Read the model definition and answer for the solid it produces. Units are mm, in the model's axes. Round coordinates to 2 decimals unless told otherwise and drop trailing zeros. Loops run counter-clockwise (first coordinate to the right, second up) from the corner with the lowest first, then second, coordinate; pieces in that order, holes last. Notation, with made-up numbers: (79.25, 5.25) -> (128.25, 5.25) arc R20 cw to (128.25, 14.25) -> close; hole circle Ø1 at (4, 11.25). An arc over 180 degrees is marked (long way). Put each result on its own line as item: value.
from build123d import *

# Parameters (mm, degrees)
BOSS_EXTRUDE1_DEPTH = 25
SKETCH2_R           = 3
CUT_EXTRUDE1_DEPTH  = 25


with BuildPart() as part:
    # Sketch1 → Boss-Extrude1 (new body, symmetric)
    with BuildSketch(Plane.XY):
        Polygon((4.75, 0), (-4.75, 0), (-11, 6.25), (-11, 7.65), (11, 7.65), (11, 6.25), align=None)
    extrude(amount=BOSS_EXTRUDE1_DEPTH, both=True)

    # Sketch2 → Cut-Extrude1 (cut, symmetric)
    with BuildSketch(Plane(origin=(0, 7.65, 0), x_dir=(1, 0, 0), z_dir=(0, 1, 0))):
        with Locations((0, 17.5)):
            Circle(SKETCH2_R)
        with Locations((0, -17.5)):
            Circle(SKETCH2_R)
    extrude(amount=CUT_EXTRUDE1_DEPTH, both=True, mode=Mode.SUBTRACT)


solid = part.part
Item 1: For a pull along X with two mould halves and no side action, classify faces 1 (the cylindrical face through (-0.65, 3.88, -14.57)), 2 (the flat face through (11, 7, 0)), 3 (the flat face through (0, 5, -25)), 4 (the flat face through (-11, 7, 0)) as pulls with the +X half, pulls with the -X half, needs draft (parallel to the pull), parting line crosses it, or undercut.
Derived:
face 1: undercut
face 2: pulls with the +X half
face 3: needs draft
face 4: pulls with the -X half
Item 2: Find the intervals of material crossed by line 1 along Z through (x, y) = (0, 2.5); line 2 along X through (y, z) = (2.75, 17.5); line 3 along X through (y, z) = (4.25, -17.5), in increasing order.
Derived:
line 1: z = -25 to -20.5, -14.5 to 14.5, 20.5 to 25
line 2: x = -7.5 to -3, 3 to 7.5
line 3: x = -9 to -3, 3 to 9
Item 3: Flat-ended cylindrical pins translate along their axes: pin 1 Ø1 at (x, y) = (-7, 2) entering from -Z; pin 2 Ø2 at (y, z) = (4.5, -8) entering from +X. Find the tip coordinate at first contact, or state that the pin passes through.
Derived:
pin 1: stops at z = -25
pin 2: stops at x = 10.25
Item 4: The part is cut by section D-D (x = 7.5). Determine the outline of the cut face in (y, z), then the cut area to 3 significant figures.
Derived:
outline: (2.75, -25) -> (7.65, -25) -> (7.65, 25) -> (2.75, 25) -> close
area: 245 mm^2
Item 5: The part is cut by section B-B (z = -17.5). Determine the outline of the cut face in (x, y).
Derived:
outline: (-11, 6.25) -> (-4.75, 0) -> (-3, 0) -> (-3, 7.65) -> (-11, 7.65) -> close; (3, 0) -> (4.75, 0) -> (11, 6.25) -> (11, 7.65) -> (3, 7.65) -> close
Item 6: The part is cut by section C-C (y = 5). Determine the outline of the cut face in (x, z), then the cut area to 3 significant figures.
Derived:
outline: (-9.75, -25) -> (9.75, -25) -> (9.75, 25) -> (-9.75, 25) -> close; hole circle Ø6 at (0, -17.5); hole circle Ø6 at (0, 17.5)
area: 918 mm^2
Item 7: The part is cut by section A-A (x = 0). Determine the outline of the cut face in (y, z).
Derived:
outline: (0, -25) -> (7.65, -25) -> (7.65, -20.5) -> (0, -20.5) -> close; (0, -14.5) -> (7.65, -14.5) -> (7.65, 14.5) -> (0, 14.5) -> close; (0, 20.5) -> (7.65, 20.5) -> (7.65, 25) -> (0, 25) -> close
